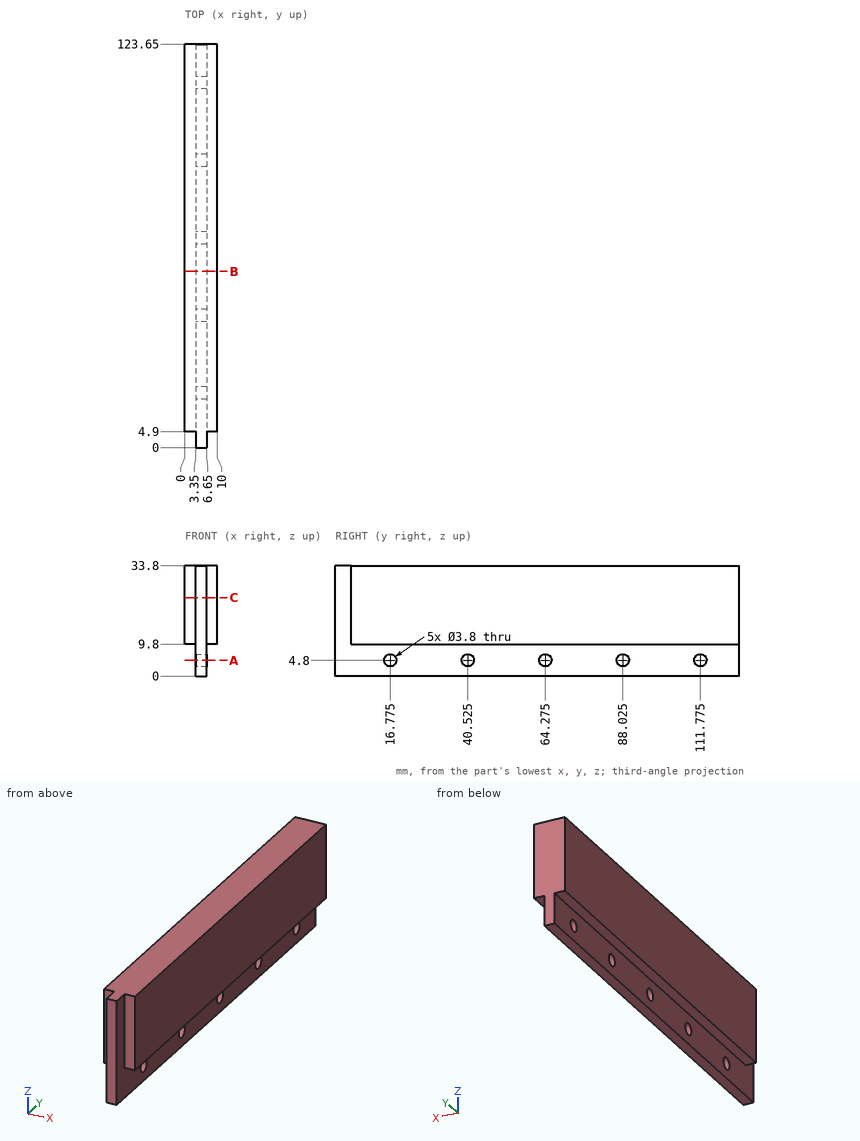
Drawing for the job (mm, zero at the part's lowest x, y, z). Give positions to 0.01 mm unless a question says otherwise; leave off trailing zeros. Write each loop counter-clockwise with the first axis right and the second up, starting at its lowest first coordinate (ties: lowest second). Pieces come first, ordered by that corner, then holes. Notation, with made-up numbers: M -29,5.25 L -22,5.25 A6 cw -22,11.25 Z; hole C 10.5,-8 d5. An arc over 180 degrees is marked long. Return JSON: item names as keys, results as strings. Group by question number.
(1) Drill centre lines: L1, parallel to Y at x = 5.6, z = 4.8 (3 decimals); L2, parallel to Z at x = 2.5, y = 66.5; L3, parallel to Y at x = 2.25, z = 16. Where is each one in solid material? Low to high. Write a range as [from, to].
(2) Flat gauge pins, fed straight in: pin 1 Ø1.5 at (x, y) = (3, 66.5) entering from -Z; pin 2 Ø1.7 at (x, y) = (1.5, 81.5) entering from -Z; pin 3 Ø5 at (y, z) = (64.275, 4.8) entering from +X; pin 4 Ø1.7 at (x, z) = (1, 25.5) entering from -Y. Where does each tip first touch, or does it go through?
(3) Band-saw the part on B-B (y = 54). Give the cut face in (x, z).
(4) Band-saw the part on C-C (z = 24). Give the cut face in (x, y).
(5) Band-saw the part on A-A (z = 4.8). Give the cut face in (x, y) (3 decimals).
Entries:
{
 "1": {"L1": "y = [0, 14.875], [18.675, 38.625], [42.425, 62.375], [66.175, 86.125], [89.925, 109.875], [113.675, 123.65]", "L2": "z = [9.8, 33.8]", "L3": "y = [4.9, 123.65]"},
 "2": {"pin 1": "stops at z = 0", "pin 2": "stops at z = 9.8", "pin 3": "stops at x = 6.65", "pin 4": "stops at y = 4.9"},
 "3": {"outline": "M 0,9.8 L 3.35,9.8 L 3.35,0 L 6.65,0 L 6.65,9.8 L 10,9.8 L 10,33.8 L 0,33.8 Z"},
 "4": {"outline": "M 0,4.9 L 3.35,4.9 L 3.35,0 L 6.65,0 L 6.65,4.9 L 10,4.9 L 10,123.65 L 0,123.65 Z"},
 "5": {"outline": "M 3.35,0 L 6.65,0 L 6.65,14.875 L 3.35,14.875 Z; M 3.35,18.675 L 6.65,18.675 L 6.65,38.625 L 3.35,38.625 Z; M 3.35,42.425 L 6.65,42.425 L 6.65,62.375 L 3.35,62.375 Z; M 3.35,66.175 L 6.65,66.175 L 6.65,86.125 L 3.35,86.125 Z; M 3.35,89.925 L 6.65,89.925 L 6.65,109.875 L 3.35,109.875 Z; M 3.35,113.675 L 6.65,113.675 L 6.65,123.65 L 3.35,123.65 Z"}
}
